Input: part model. Units: mm. Frame: model coordinates. A direction names the side the tool comes from. Coordinates: 2 decimals unless noted, no trailing zeros. Order: outer loops, then holes, each group sorted by start corner. A loop starts at its lowest first (then second) coordinate and runs counter-clockwise, first axis right, second up. Notation, with made-up numbers: M 36,84 L 69,84 A28 ccw 69,116 Z; hole C -8.75,37.25 d5. An arc over 180 degrees is marked long. Answer in a Markdown table with one row per item.
from build123d import *

# Parameters (mm, degrees)
F0_R     = 3.175
F1_DEPTH = 6.35
F2_R     = 5.3594
F3_DEPTH = 0.7874
F4_R     = 5.3594
F5_DEPTH = 2.3876
F6_R     = 1.778
F8_DEPTH = 2.8194


with BuildPart() as f1:
    # F0 (on Top) → F1 (new body)
    with BuildSketch(Plane.XY):
        Circle(F0_R)
    extrude(amount=F1_DEPTH)

    # F2 (on face) → F3 (join)
    with BuildSketch(Plane.XY.offset(6.35)):
        Circle(F2_R)
    extrude(amount=F3_DEPTH)

    # F4 (on face) → F5 (join)
    with BuildSketch(Plane.XY.offset(7.1374)):
        Circle(F4_R)
    extrude(amount=F5_DEPTH)

    # F6
    f6_edges = [f1.edges().sort_by_distance(p)[0] for p in [
        (-5.3594, 0, 9.525),
    ]]
    fillet(f6_edges, radius=F6_R)

    # F7 (on face) → F8 (cut)
    with BuildSketch(Plane.XY.offset(9.525)):
        Polygon((1.1065416167, -2.0003403837), (2.2856163968, -0.0418770414), (1.1790747801, 1.9584633423), (-1.1065416167, 2.0003403837), (-2.2856163968, 0.0418770414), (-1.1790747801, -1.9584633423), align=None)
    extrude(amount=-F8_DEPTH, mode=Mode.SUBTRACT)


solid = f1.part
1) Cut plane A-A, the plane x = 0. Output: boundary loops of the cut face in (y, z) (3 decimals).
Resolved:
| item | result |
|---|---|
| outline | M -5.359,6.35 L -3.175,6.35 L -3.175,0 L 3.175,0 L 3.175,6.35 L 5.359,6.35 L 5.359,7.747 A1.778 ccw 3.581,9.525 L 1.98,9.525 L 1.98,6.706 L -1.98,6.706 L -1.98,9.525 L -3.581,9.525 A1.778 ccw -5.359,7.747 Z |
2) Contact query for flat-ended pins moving along their axis: pin 1 (3 mm diameter, centred on x = -4, y = -4, fed in from -Z); pin 2 (5 mm diameter, centred on y = 4, z = 2, fed in from -X); pin 3 (1 mm diameter, centred on x = 3.5, z = 8.5, fed in from -Y). Output: stop coordinate, or through.
Resolved:
| item | result |
|---|---|
| pin 1 | stops at z = 6.35 |
| pin 2 | stops at x = -2.8 |
| pin 3 | stops at y = -4.31 |
3) Mould query, pull axis X, two halves, no side actions, for faces 1 (the face through (0, 0, 0)), 2 (the face through (1.74, 0.944, 8.135)), 3 (the face through (-0.69, -3.1, 3.13)). Classes: +X half, -X half, draft (parallel to the pull), parting line (faces both ways), or undercut.
Resolved:
| item | result |
|---|---|
| face 1 | draft |
| face 2 | undercut |
| face 3 | parting line |
4) Reachability of faces 4 (the face through (-0.1, -3.5, 6.35)), 5 (the face through (1.69, -1.03, 8.14)), 6 (the face through (2, -2, 9.525)) from +Z, -Z, +X, -X, +Y, -Y: full face, straight path, thin tool, end or side. Return the list, or none.
Resolved:
| item | result |
|---|---|
| face 4 | -Z |
| face 5 | +Z |
| face 6 | +Z, +X, -X, +Y, -Y |
5) Material intervals for probe 1 along X at (y, z) = (2.5, 2); probe 2 along Z at (x, y) = (0.5, -0.25), sorted ascending.
Resolved:
| item | result |
|---|---|
| probe 1 | x = -1.96 to 1.96 |
| probe 2 | z = 0 to 6.71 |
